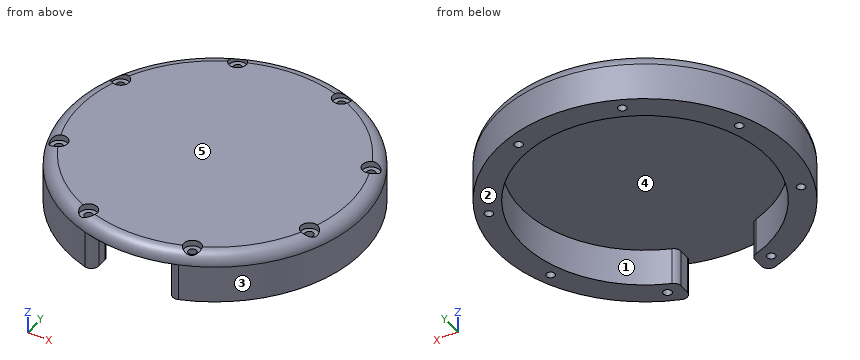
from build123d import *

# Parameters (mm, degrees)
SALIENTE_EXTRUIR1_DEPTH                              = 15
CROQUIS2_R                                           = 60
SALIENTE_EXTRUIR2_DEPTH                              = 5
REFRENTADO_PARA_TORNILLO_CON_CABEZA_TRON_D           = 3.4
REFRENTADO_PARA_TORNILLO_CON_CABEZA_TRON_CBORE_D     = 7
REFRENTADO_PARA_TORNILLO_CON_CABEZA_TRON_CBORE_DEPTH = 2.4
REDONDEO1_R                                          = 5


with BuildPart() as part:
    # Croquis1 → Saliente-Extruir1 (new body)
    with BuildSketch(Plane.XY):
        with BuildLine():
            Line((-15, -49.849774322), (-15, -54.083269132))
            ThreePointArc((-15, -54.083269132), (-16.245307044, -56.516590449), (-18.947368421, -56.929756981))
            ThreePointArc((-18.947368421, -56.929756981), (0, 60), (18.947368421, -56.929756981))
            ThreePointArc((18.947368421, -56.929756981), (16.245307044, -56.516590449), (15, -54.083269132))
            Line((15, -54.083269132), (15, -49.849774322))
            ThreePointArc((15, -49.849774322), (15.544739955, -48.125912926), (16.981132075, -47.028088983))
            ThreePointArc((16.981132075, -47.028088983), (0, 50), (-16.981132075, -47.028088983))
            ThreePointArc((-16.981132075, -47.028088983), (-15.544739955, -48.125912926), (-15, -49.849774322))
        make_face()
    extrude(amount=SALIENTE_EXTRUIR1_DEPTH)

    # Croquis2 → Saliente-Extruir2 (add)
    with BuildSketch(Plane.XY.offset(15)):
        with Locations(Location((0, 0, 0), (0, 0, 251.591519829))):
            Circle(CROQUIS2_R)
    extrude(amount=SALIENTE_EXTRUIR2_DEPTH)

    # Refrentado para tornillo con cabeza troncocónica de M31 (through all)
    with Locations(Plane.XY.offset(20)):
        with Locations((-21.04758878, 50.813374288), (21.04758878, 50.813374288), (50.813374288, 21.04758878), (50.813374288, -21.04758878), (21.04758878, -50.813374288), (-21.04758878, -50.813374288), (-50.813374288, -21.04758878), (-50.813374288, 21.04758878)):
            CounterBoreHole(REFRENTADO_PARA_TORNILLO_CON_CABEZA_TRON_D / 2, REFRENTADO_PARA_TORNILLO_CON_CABEZA_TRON_CBORE_D / 2, REFRENTADO_PARA_TORNILLO_CON_CABEZA_TRON_CBORE_DEPTH)

    # Redondeo1
    # the kernel refuses this fillet: 5 mm, written as the material it takes off along each edge
    with BuildSketch(Plane(origin=(0, 0, 20), x_dir=(-0.31578947369106963, -0.9488292830145564, 0), z_dir=(-0.9488292830145564, 0.31578947369106963, 0))) as redondeo1_piece_1:
        with BuildLine():
            CenterArc((60 - REDONDEO1_R, -REDONDEO1_R), REDONDEO1_R, 0, 90)
            Line((60 - REDONDEO1_R, 0), (60, 0))
            Line((60, 0), (60, -REDONDEO1_R))
        make_face()
    revolve(axis=Axis((0, 0, 20), (0, 0, 1)), mode=Mode.SUBTRACT)


solid = part.part
Design review of the part built by this model. Coordinates are the model's own, in mm. Face numbers are marked on the shaded views. A direction names the side the tool comes from. Give positions to 0.01 mm unless a question says otherwise; leave off trailing zeros. Loops run counter-clockwise (first coordinate to the right, second up) from the corner with the lowest first, then second, coordinate; pieces in that order, holes last. Notation, with made-up numbers: (65.25, 25) - (113.25, 25) arc R29 ccw to (113.25, 55) - close; hole circle Ø5 at (1.25, 45). An arc over 180 degrees is marked (long way). Use CSV: the item, a comma, the result in double quotes. Start each with the question number.
1. Draft analysis for pull direction X (two halves, no side actions). For the marked faces 3, 4 and 5, state which applies: released by +X, released by -X, zero draft, split by the parting line, or undercut.
2. Insertion check: P1, Ø2, axis at y = -24.5, z = 5.5, coming from the -X side; P2, Ø6, axis at x = 46, z = 6, coming from the -Y side; P3, Ø1.3, axis at y = -51.5, z = 11, coming from the +X side. Each pin has a flat end and moves straight along its axis. Give the tip position at first contact, or say it passes through.
3. Add section C-C (x = 0). State the section outline as (y, z) points, plus the area to 3 significant figures.
4. Add section A-A (y = 0). State the section outline as (x, z) points, plus the area to 3 significant figures.
5. Machinability: for the marked faces 1 and 2, which of the approach directions +Z, -Z, +X, -X, +Y, -Y give a long, thin tool a straight path to every point of the face, cutting with its end or side? Answer none if there is none.
6. Wall thickness on L1, parallel to X at y = -51.5, z = 6.5; L2, parallel to X at y = 0, z = 4.5; L3, parallel to Z at x = 1, y = -46.5: over which ranges is each line inside the solid? List them lowest first.
7. Add section B-B (z = 3.25). Count the separate pieces of the cut face and the enclosed holes in it, plus the area to 3 significant figures.
Results found:
1,face 3,"split by the parting line"
1,face 4,"undercut"
1,face 5,"zero draft"
2,P1,"stops at x = -55.21"
2,P2,"stops at y = -41.84"
2,P3,"stops at x = 31.85"
3,outline,"(-60, 15) - (50, 15) - (50, 0) - (60, 0) - (60, 15) arc R5 ccw to (55, 20) - (-55, 20) arc R5 ccw to start"
3,area,"739 mm²"
4,outline,"(-60, 0) - (-50, 0) - (-50, 15) - (50, 15) - (50, 0) - (60, 0) - (60, 15) arc R5 ccw to (55, 20) - (-55, 20) arc R5 ccw to (-60, 15) - close"
4,area,"889 mm²"
5,face 1,"-Z"
5,face 2,"-Z, +X, -X, +Y, -Y"
6,L1,"x = -30.79 to -22.6, -19.49 to -15, 15 to 19.49, 22.6 to 30.79"
6,L2,"x = -60 to -50, 50 to 60"
6,L3,"z = 15 to 20"
7,separate pieces,"1"
7,enclosed holes,"8"
7,area,"3,070 mm²"
